Model file for the job. Use its own axes, mm. Give positions to 0.01 mm unless a question says otherwise; leave off trailing zeros. Return JSON: item names as keys, results as strings. Group by question number.
1. Two-plate mould, pull along Y, no slides. Class faces 1 (the face through (6, 15, 0)), 2 (the face through (-3, 5, 0)), 3 (the face through (1.4, 25, 1.4)): released by +Y, released by -Y, zero draft, split by the parting line, or undercut.
2. Pin check, flat tips, straight feed: pin 1 (6 mm diameter, centred on y = -441.5, z = 4.5, fed in from -X); pin 2 (5.5 mm diameter, centred on x = 0.5, z = 0, fed in from -Y); pin 3 (6 mm diameter, centred on x = 2, z = 1, fed in from +Y). Stop position of each tip, or through.
3. Wall check: probe 1 along Y at (x, z) = (-4.5, -3.75); probe 2 along X at (y, z) = (49.5, -1); probe 3 along Y at (x, z) = (74, -0.75). Give the ranges that are in metal, low to high. Write a range as [from, to].
Autodesk Inventor part; units mm, degrees
ref_plane "YZ Plane" through (0, 0, 0) normal (1, 0, 0) x (0, 1, 0)
ref_plane "XZ Plane" through (0, 0, 0) normal (0, 1, 0) x (-1, 0, 0)
ref_plane "XY Plane" through (0, 0, 0) normal (0, 0, 1) x (1, 0, 0)
sketch "Sketch1" plane through (0, 0, 0) normal (0, 0, 1) x (1, 0, 0)
  line L0 (-7.2, 0) -> (1.2, 0) construction
  line L1 (0, -5) -> (0, 30) construction
  line L2 (0, 0) -> (-2.5, 0)
  line L3 (-2.5, 0) -> (-2.5, 5)
  line L4 (-2.5, 5) -> (-6, 5)
  line L5 (-6, 5) -> (-6, 25)
  line L6 (-6, 25) -> (0, 25)
  line L7 (0, 25) -> (0, 0)
  dimension "d0" = 5
  dimension "d1" = 12
  dimension "d2" = 5
  dimension "d3" = 25
revolve "Revolution1" add sketch "Sketch1" angle 360 about axis through (0, -10, 0) along (0, 1, 0)
sketch "Sketch2" plane through (0, 0, 0) normal (0, 0, 1) x (1, 0, 0)
  line L0 (0, -5) -> (0, 30) construction
  line L1 (6, 25) -> (-6, 25) construction
  line L2 (0, 25) -> (0, 30)
  line L3 (105.9337, -600) -> (105.9337, 80)
  arc A0 (105.9337, 80) -> (-4.9943, 46.5746) centre (45.4337, 80) ccw
  arc A1 (0, 30) -> (-4.9943, 46.5746) centre (-30, 30) ccw
  line L4 (-74.1691, 0) -> (235.0145, 0)
  point P0 (0, 0)
  point P1 (0, 40.0497)
  dimension "d5" = 30
  dimension "d9" = 5
  dimension "d10" = 60.5
  dimension "d11" = 80
  dimension "d12" = 600
sketch "Sketch3" plane through (0, 25, 0) normal (0, 1, 0) x (1, 0, 0)
  circle A0 centre (0, 0) radius 1.75
  dimension "d6" = 3.5
sweep "Sweep1" add profiles "Sketch3" path "Sketch2" path curves L2 A1 A0 L3
properties part number "F118Laser"
Result:
{
 "1": {"face 1": "zero draft", "face 2": "released by -Y", "face 3": "undercut"},
 "2": {"pin 1": "stops at x = 105.03", "pin 2": "stops at y = 0", "pin 3": "stops at y = 127.23"},
 "3": {"probe 1": "y = [5, 25]", "probe 2": "x = [-8.47, -5.15], [104.5, 107.37]", "probe 3": "y = [131.53, 135.12]"}
}
